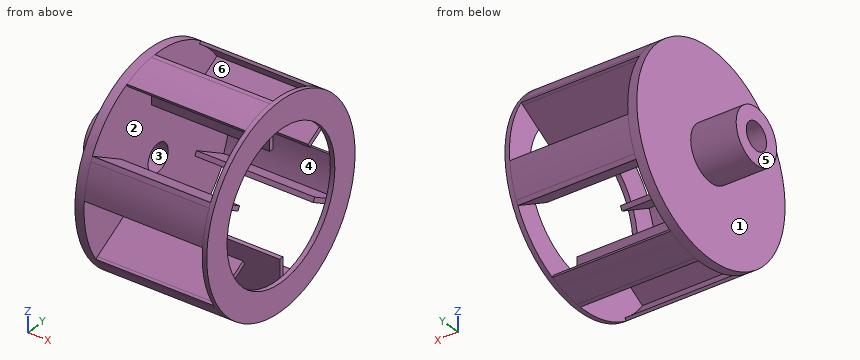
```python
from build123d import *

# Parameters (mm, degrees)
SKETCH3_R           = 38.1
SKETCH3_R_2         = 19.05
BOSS_EXTRUDE1_DEPTH = 76.2
SKETCH3_3_R         = 139.7
SKETCH3_3_R_2       = 38.1
BOSS_EXTRUDE2_DEPTH = 12.7
BOSS_EXTRUDE5_START = 165.1
BOSS_EXTRUDE5_DEPTH = 165.1
CIRPATTERN1_COUNT   = 6
BOSS_EXTRUDE6_START = 6.35
SKETCH5_R           = 139.7
SKETCH5_R_2         = 101.6
BOSS_EXTRUDE6_DEPTH = 6.35


with BuildPart() as part:
    # Sketch3 → Boss-Extrude1 (new body)
    with BuildSketch(Plane(origin=(0, 0, 0), x_dir=(0, 0, -1), z_dir=(1, 0, 0))):
        Circle(SKETCH3_R)
        Circle(SKETCH3_R_2, mode=Mode.SUBTRACT)
    extrude(amount=-BOSS_EXTRUDE1_DEPTH)

    # Sketch3_3 → Boss-Extrude2 (add)
    with BuildSketch(Plane(origin=(0, 0, 0), x_dir=(0, 0, -1), z_dir=(1, 0, 0))):
        Circle(SKETCH3_3_R)
        Circle(SKETCH3_3_R_2, mode=Mode.SUBTRACT)
    extrude(amount=-BOSS_EXTRUDE2_DEPTH)

    # Sketch4_4 → Boss-Extrude5 (add)
    with BuildSketch(Plane(origin=(0, 0, 0), x_dir=(0, 0, -1), z_dir=(1, 0, 0)).offset(BOSS_EXTRUDE5_START)):
        with BuildLine():
            Line((-49.098522628, 59.641135768), (-43.599261314, 62.816135768))
            Line((-43.599261314, 62.816135768), (-73.370038531, 114.380634489))
            ThreePointArc((-73.370038531, 114.380634489), (-76.028948152, 112.630773517), (-78.646142874, 110.819115278))
            Line((-78.646142874, 110.819115278), (-49.098522628, 59.641135768))
        make_face()
        with BuildLine():
            ThreePointArc((-111.366656278, 77.868863928), (-96.424300498, 95.752004541), (-78.646142874, 110.819115278))
            Line((-78.646142874, 110.819115278), (-80.559287431, 114.132778852))
            ThreePointArc((-80.559287431, 114.132778852), (-98.883164233, 98.682368391), (-114.296295848, 80.32712341))
            Line((-114.296295848, 80.32712341), (-111.366656278, 77.868863928))
        make_face()
        with BuildLine():
            ThreePointArc((-78.646142874, 110.819115278), (-76.028948152, 112.630773517), (-73.370038531, 114.380634489))
            Line((-73.370038531, 114.380634489), (-75.277064912, 117.683701073))
            ThreePointArc((-75.277064912, 117.683701073), (-77.938401575, 115.938326536), (-80.559287431, 114.132778852))
            Line((-80.559287431, 114.132778852), (-78.646142874, 110.819115278))
        make_face()
    boss_extrude5 = extrude(amount=-BOSS_EXTRUDE5_DEPTH)

    # CirPattern1: Boss-Extrude5 ×6 about axis
    cirpattern1_axis = Axis((0, 0, 0), (1, 0, 0))
    for i in range(1, CIRPATTERN1_COUNT):
        add(boss_extrude5.rotate(cirpattern1_axis, i * 360 / CIRPATTERN1_COUNT))

    # Sketch5 → Boss-Extrude6 (add)
    with BuildSketch(Plane(origin=(165.1, 0, 0), x_dir=(0, 0, -1), z_dir=(1, 0, 0)).offset(BOSS_EXTRUDE6_START)):
        Circle(SKETCH5_R)
        with Locations(Location((0, 0, 0), (0, 0, 183.583321698))):
            Circle(SKETCH5_R_2, mode=Mode.SUBTRACT)
    extrude(amount=-BOSS_EXTRUDE6_DEPTH)


solid = part.part
```
Could you check a few things on this model? Use its own coordinates, in mm. Face numbers are marked on the shaded views. A direction names the side the tool comes from. Coordinates: 2 decimals unless noted, no trailing zeros. Loops run counter-clockwise (first coordinate to the right, second up) from the corner with the lowest first, then second, coordinate; pieces in that order, holes last. Notation, with made-up numbers: M -4.75,-16 L 22.25,-16 A13 ccw 22.25,8 Z; hole C -19.75,81 d11. An arc over 180 degrees is marked long. Put each result on its own line as item: value. Start each with the question number.
(1) Suppose I cut it at C-C on z = 86. Please give me the cut outline in (x, y).
(2) Suppose I cut it at D-D on x = -57.5. Please give me the cut outline in (y, z), then the cut area to 3 significant figures.
(3) Will these pins go through, and if not, where does the flat tip stop? P1, Ø6, axis at y = 81, z = 45, coming from the -X side; P2, Ø5, axis at x = 52, y = -11, coming from the -Z side; P3, Ø5.5, axis at y = -81.5, z = 37, coming from the +X side.
(4) Thinking about a two-plate mould opening in Z: for the marked faces 4, 5 and 6, which applies, pulls with the +Z half, pulls with the -Z half, needs draft (parallel to the pull), parting line crosses it, or undercut?
(5) For the marked faces 1, 2 and 3, which set-ups out of +Z, -Z, +X, -X, +Y, -Y let a thin tool reach every point of the face, with its end or its side?
(6) I need wall thicknesses on line 1 (Z direction, x = 167.75, y = 0); line 2 (Y direction, x = -24.5, z = 0). Which ranges of each line are inside material? Lowest first, please. Write a range as from..to.
(7) Suppose I cut it at A-A on y = 0. Please give me the cut outline in (x, z), then the cut area to 3 significant figures.
Solutions:
1. outline: M -12.7,-110.09 L 0,-110.09 L 0,-12.7 L 165.1,-12.7 L 165.1,-6.35 L 0,-6.35 L 0,105.21 L 165.1,105.21 L 165.1,54.1 L 171.45,54.1 L 171.45,110.09 L -12.7,110.09 Z; M 165.1,-110.09 L 171.45,-110.09 L 171.45,-54.1 L 165.1,-54.1 Z
2. outline: C 0,0 d76.2; hole C 0,0 d38.1
2. area: 3,420 mm2
3. P1: stops at x = -12.7
3. P2: stops at z = 76.2
3. P3: stops at x = 165.1
4. face 4: pulls with the +Z half
4. face 5: needs draft
4. face 6: undercut
5. face 1: -X
5. face 2: none
5. face 3: +X, -X
6. line 1: z = -139.7..-101.6, 101.6..139.7
6. line 2: y = -38.1..-19.05, 19.05..38.1
7. outline: M -76.2,-38.1 L -12.7,-38.1 L -12.7,-139.7 L 0,-139.7 L 0,-19.05 L -76.2,-19.05 Z; M -76.2,19.05 L 0,19.05 L 0,139.7 L -12.7,139.7 L -12.7,38.1 L -76.2,38.1 Z; M 165.1,-139.7 L 171.45,-139.7 L 171.45,-101.6 L 165.1,-101.6 Z; M 165.1,101.6 L 171.45,101.6 L 171.45,139.7 L 165.1,139.7 Z
7. area: 5,970 mm2
